from build123d import *

# Parameters (mm, degrees)
F0_R     = 4
F1_DEPTH = 5
F2_R     = 3.226703
F3_DEPTH = 1
F4_R     = 1
F5_DEPTH = 4.001


with BuildPart() as f1:
    # F0 (on Top) → F1 (new body)
    with BuildSketch(Plane.XY):
        Circle(F0_R)
    extrude(amount=F1_DEPTH)

    # F2 (on face) → F3 (cut)
    with BuildSketch(Plane.XY.offset(5)):
        Circle(F2_R)
    extrude(amount=-F3_DEPTH, mode=Mode.SUBTRACT)

    # F4 (on face) → F5 (cut, through all)
    with BuildSketch(Plane.XY.offset(4)):
        Circle(F4_R)
    extrude(amount=-F5_DEPTH, mode=Mode.SUBTRACT)


solid = f1.part
For this review, take the finished solid that the model builds, in its own axes (mm). A direction names the side the tool comes from. Round coordinates to 2 decimals unless told otherwise and drop trailing zeros. Order: outer loops, then holes, each group sorted by start corner. A loop starts at its lowest first (then second) coordinate and runs counter-clockwise, first axis right, second up. Notation, with made-up numbers: M 22.25,-14 L 52.25,-14 A10 cw 52.25,-10 Z; hole C 69,80.5 d5. An arc over 180 degrees is marked long. Write each question's results on one line, items separated by ' | '. Start each with the question number.
1. Draft analysis for pull direction Y (two halves, no side actions). For faces 1 (the face through (-0.867, -3.905, 2.465)), 2 (the face through (1, -1, 0)), 3 (the face through (1, 1, 4)), 4 (the face through (0, -1, 2)), state which applies: pulls with the +Y half, pulls with the -Y half, needs draft (parallel to the pull), parting line crosses it, or undercut.
2. Add section D-D (x = 1.75). State the section outline as (y, z) points, then the cut area to 3 significant figures.
3. To check wall thickness, follow L1, parallel to Y at x = 0, z = 4.3; L2, parallel to Z at x = -0.25, y = 2.75; L3, parallel to X at y = 1.75, z = 4.4. State the ranges of each line that lie inside material, in increasing order. Write a range as [from, to].
4. Add section A-A (y = 0). State the section outline as (x, z) points.
5. Tool access review of faces 5 (the face through (-0.4, 3.2, 4.5)), 6 (the face through (-3, 2, 5)): name each direction out of +Z, -Z, +X, -X, +Y, -Y from which nothing blocks a thin tool from reaching the whole face with its end or side.
6. Clearance check with flat-ended pins moving along their axes: pin 1 Ø4 at (x, y) = (0.5, 1.5) entering from +Z; pin 2 Ø3 at (x, y) = (0, 0) entering from +Z; pin 3 Ø1.5 at (x, z) = (3, 4) entering from -Y. State where each tip first meets the part, or that it passes through.
7. Add section C-C (z = 2.55). State the section outline as (x, y) points, then the cut area to 3 significant figures.
Output values:
1) face 1: parting line crosses it | face 2: needs draft | face 3: undercut | face 4: undercut
2) outline: M -3.6,0 L 3.6,0 L 3.6,5 L 2.71,5 L 2.71,4 L -2.71,4 L -2.71,5 L -3.6,5 Z | area: 30.5 mm^2
3) L1: [-4, -3.23], [3.23, 4] | L2: [0, 4] | L3: [-3.6, -2.71], [2.71, 3.6]
4) outline: M -4,0 L -1,0 L -1,4 L -3.23,4 L -3.23,5 L -4,5 Z; M 1,0 L 4,0 L 4,5 L 3.23,5 L 3.23,4 L 1,4 Z
5) face 5: +Z | face 6: +Z, +X, -X, +Y, -Y
6) pin 1: z = 5 | pin 2: z = 4 | pin 3: y = -3.31
7) outline: C 0,0 d8; hole C 0,0 d2 | area: 47.1 mm^2
